```python
from build123d import *

# Parameters (mm, degrees)
SKETCH1_W           = 3
SKETCH1_H           = 60
BOSS_EXTRUDE1_DEPTH = 250
FILLET1_R           = 10
FILLET2_R           = 10
SKETCH2_R           = 4.25
CUT_EXTRUDE1_DEPTH  = 4
SKETCH9_R           = 7.8
CUT_EXTRUDE7_DEPTH  = 4
SKETCH11_R          = 7.8
CUT_EXTRUDE8_DEPTH  = 4
SKETCH13_R          = 2
CUT_EXTRUDE9_DEPTH  = 4
CUT_EXTRUDE13_DEPTH = 10
FILLET3_R           = 2
FILLET4_R           = 1
SKETCH18_R          = 1.5
SKETCH18_R_2        = 1.499999992
CUT_EXTRUDE15_DEPTH = 4
CUT_EXTRUDE16_DEPTH = 4


with BuildPart() as part:
    # Sketch1 → Boss-Extrude1 (new body)
    with BuildSketch(Plane.XY):
        Rectangle(SKETCH1_W, SKETCH1_H)
    extrude(amount=BOSS_EXTRUDE1_DEPTH)

    # Fillet1
    fillet1_edges = [part.edges().sort_by_distance(p)[0] for p in [
        (0, 30, 250),
    ]]
    fillet(fillet1_edges, radius=FILLET1_R)

    # Fillet2
    fillet2_edges = [part.edges().sort_by_distance(p)[0] for p in [
        (0, -30, 250),
    ]]
    fillet(fillet2_edges, radius=FILLET2_R)

    # Sketch2 → Cut-Extrude1 (cut, through all)
    with BuildSketch(Plane.ZY.offset(1.5)):
        with Locations((230, 0)):
            Circle(SKETCH2_R)
    extrude(amount=-CUT_EXTRUDE1_DEPTH, mode=Mode.SUBTRACT)

    # Sketch9 → Cut-Extrude7 (cut, through all)
    with BuildSketch(Plane(origin=(1.5, 0, 0), x_dir=(0, 0, -1), z_dir=(1, 0, 0))):
        with Locations((-230, 0)):
            Circle(SKETCH9_R)
    extrude(amount=-CUT_EXTRUDE7_DEPTH, mode=Mode.SUBTRACT)

    # Sketch11 → Cut-Extrude8 (cut, through all)
    with BuildSketch(Plane.ZY.offset(1.5)):
        with Locations((73, -7)):
            Circle(SKETCH11_R)
    extrude(amount=-CUT_EXTRUDE8_DEPTH, mode=Mode.SUBTRACT)

    # Sketch13 → Cut-Extrude9 (cut, through all)
    with BuildSketch(Plane(origin=(1.5, 0, 0), x_dir=(0, 0, -1), z_dir=(1, 0, 0))):
        with Locations((-87, 22)):
            Circle(SKETCH13_R)
        with Locations((-59, 22)):
            Circle(SKETCH13_R)
        with Locations((-59, -18)):
            Circle(SKETCH13_R)
        with Locations((-87, -18)):
            Circle(SKETCH13_R)
    extrude(amount=-CUT_EXTRUDE9_DEPTH, mode=Mode.SUBTRACT)

    # Sketch16 → Cut-Extrude13 (cut)
    with BuildSketch(Plane(origin=(1.5, 0, 0), x_dir=(0, 0, -1), z_dir=(1, 0, 0))):
        Polygon((-146.788564399, 27.2), (-174.288564399, 27.2), (-146.788564399, 4.184615385), align=None)
        Polygon((-109.288564399, 27.2), (-136.788564399, 27.2), (-136.788564399, 4.184615385), align=None)
        Polygon((-114, -17.994443239), (-114, 18.25689082), (-134.959973954, 0.715004926), align=None)
        Polygon((-148.617154843, 0.715004926), (-171.981755255, 20.269378193), (-171.981755255, -20.140878829), align=None)
        Polygon((-109.288564399, -27.2), (-138.721101597, -2.567230406), (-138.721101597, -27.2), align=None)
        Polygon((-144.856027201, -2.567230406), (-174.288564399, -27.2), (-144.856027201, -27.2), align=None)
    extrude(amount=-CUT_EXTRUDE13_DEPTH, mode=Mode.SUBTRACT)

    # Fillet3
    fillet3_edges = [part.edges().sort_by_distance(p)[0] for p in [
        (0, 0.715004926, 134.959973954),
        (0, -2.567230406, 144.856027201),
        (0, 4.184615385, 146.788564399),
        (0, -2.567230406, 138.721101597),
        (0, 0.715004926, 148.617154843),
        (0, 4.184615385, 136.788564399),
    ]]
    fillet(fillet3_edges, radius=FILLET3_R)

    # Fillet4
    fillet4_edges = [part.edges().sort_by_distance(p)[0] for p in [
        (0, 18.25689082, 114),
        (0, -17.994443239, 114),
        (0, -27.2, 174.288564399),
        (0, 27.2, 174.288564399),
        (0, -27.2, 109.288564399),
        (0, 20.269378193, 171.981755255),
        (0, -20.140878829, 171.981755255),
        (0, 27.2, 109.288564399),
    ]]
    fillet(fillet4_edges, radius=FILLET4_R)

    # Sketch18 → Cut-Extrude15 (cut, through all)
    with BuildSketch(Plane.ZY.offset(1.5)):
        with Locations((182.288564399, 24.750000007)):
            Circle(SKETCH18_R)
        with Locations((182.288564399, 7e-09)):
            Circle(SKETCH18_R)
        with Locations((182.288564399, -24.749999993)):
            Circle(SKETCH18_R)
        with Locations((28.351822221, 24.750000005)):
            Circle(SKETCH18_R_2)
        with Locations((28.351822214, 0)):
            Circle(SKETCH18_R)
        with Locations((28.351822221, -24.749999995)):
            Circle(SKETCH18_R_2)
    extrude(amount=-CUT_EXTRUDE15_DEPTH, mode=Mode.SUBTRACT)

    # Sketch22 → Cut-Extrude16 (cut, through all)
    with BuildSketch(Plane(origin=(1.5, 0, 0), x_dir=(0, 0, -1), z_dir=(1, 0, 0))):
        with BuildLine():
            Line((-140.3152575, 16.383557477), (-140.3152575, 0.290513908))
            ThreePointArc((-140.3152575, 0.290513908), (-141.8152575, -1.209486092), (-143.3152575, 0.290513908))
            Line((-143.3152575, 0.290513908), (-143.3152575, 16.383557477))
            ThreePointArc((-143.3152575, 16.383557477), (-141.8152575, 17.883557477), (-140.3152575, 16.383557477))
        make_face()
    extrude(amount=-CUT_EXTRUDE16_DEPTH, mode=Mode.SUBTRACT)


solid = part.part
```
Geometry check sheet. Reference: the model listing, model coordinates, mm. A direction names the side the tool comes from. Coordinates: 2 decimals unless noted, no trailing zeros. Order: outer loops, then holes, each group sorted by start corner. A loop starts at its lowest first (then second) coordinate and runs counter-clockwise, first axis right, second up. Notation, with made-up numbers: M -17.5,-10.5 L 15.5,-10.5 A22 cw 15.5,15.5 Z; hole C -37.5,2 d1. An arc over 180 degrees is marked long. One line per question, with ' | ' between items. Start each with the question number.
Item 1: Cross-section at B-B on y = 11.5. Enter the section's corners in (x, z), then the cut area to 3 significant figures.
Item 2: Cross-section at C-C on z = 127. Enter the section's corners in (x, y).
Item 3: Cross-section at A-A on z = 73. Enter the section's corners in (x, y), then the cut area to 3 significant figures.
Item 4: Cross-section at D-D on x = 0.25. State how many separate pieces and enclosed holes the cut face has, then the cut area to 3 significant figures.
Item 5: Gauge pin test, flat end, axial feed: pin 1 (18 mm diameter, centred on y = 0, z = 230, fed in from +X). Record the tip position at first contact, or that the pin passes through.
Item 6: Material ranges on L1, parallel to Y at x = -0.8, z = 59; L2, parallel to Y at x = -0.4, z = 57.5; L3, parallel to Z at x = 0.55, y = 24.5, recorded low to high. Write a range as [from, to].
Item 7: Set-up check for faces 1 (the cylindrical face through (0.02, -26.99, 247.15)), 2 (the flat face through (0.021, 10.431, 160.226)): record each of +Z, -Z, +X, -X, +Y, -Y from which the full face is reachable in a straight line by a thin tool's end or side.
Item 8: Draft check along Y on faces 3 (the flat face through (1.5, -14, 123)), 4 (the flat face through (0.02, 16.05, 122.61)), 5 (the cylindrical face through (0.02, 27.15, 246.99)). Enter one of: pulls with the +Y half, pulls with the -Y half, needs draft (parallel to the pull), parting line crosses it, or undercut.
Findings:
1) outline: M -1.5,0 L 1.5,0 L 1.5,114 L -1.5,114 Z; M -1.5,122.07 L 1.5,122.07 L 1.5,128.05 L -1.5,128.05 Z; M -1.5,136.79 L 1.5,136.79 L 1.5,140.32 L -1.5,140.32 Z; M -1.5,143.32 L 1.5,143.32 L 1.5,146.79 L -1.5,146.79 Z; M -1.5,155.53 L 1.5,155.53 L 1.5,161.5 L -1.5,161.5 Z; M -1.5,171.98 L 1.5,171.98 L 1.5,250 L -1.5,250 Z | area: 633 mm²
2) outline: M -1.5,-30 L 1.5,-30 L 1.5,-27.2 L -1.5,-27.2 Z; M -1.5,-12.38 L 1.5,-12.38 L 1.5,-6.39 L -1.5,-6.39 Z; M -1.5,7.38 L 1.5,7.38 L 1.5,12.38 L -1.5,12.38 Z; M -1.5,27.2 L 1.5,27.2 L 1.5,30 L -1.5,30 Z
3) outline: M -1.5,-30 L 1.5,-30 L 1.5,-14.8 L -1.5,-14.8 Z; M -1.5,0.8 L 1.5,0.8 L 1.5,30 L -1.5,30 Z | area: 133 mm²
4) separate pieces: 1 | enclosed holes: 19 | area: 12,200 mm²
5) pin 1: stops at x = 1.5
6) L1: y = [-30, -20], [-16, 20], [24, 30] | L2: y = [-30, -19.32], [-16.68, 20.68], [23.32, 30] | L3: z = [0, 26.87], [29.83, 112.51], [136.79, 146.79], [171.06, 180.81], [183.77, 248.93]
7) face 1: +Z, +X, -X, -Y | face 2: +X, -X
8) face 3: needs draft | face 4: undercut | face 5: pulls with the +Y half
